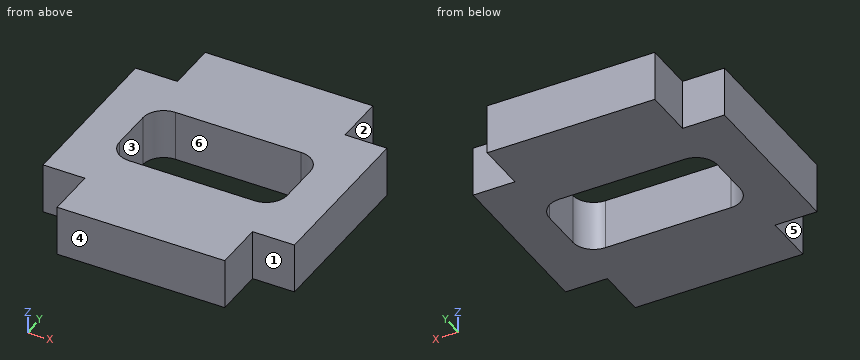
from build123d import *

# Parameters (mm, degrees)
SALIENTE_EXTRUIR1_DEPTH = 3


with BuildPart() as part:
    # Croquis1 → Saliente-Extruir1 (new body)
    with BuildSketch(Plane.XY):
        Polygon((-5, -8), (5, -8), (5, -5), (7.5, -5), (7.5, 5), (5, 5), (5, 8), (-5, 8), (-5, 5), (-7.5, 5), (-7.5, -5), (-5, -5), align=None)
        with BuildLine():
            ThreePointArc((5, -1.25), (4.633883476, -2.133883476), (3.75, -2.5))
            Line((3.75, -2.5), (-3.75, -2.5))
            ThreePointArc((-3.75, -2.5), (-4.633883476, -2.133883476), (-5, -1.25))
            Line((-5, -1.25), (-5, 1.25))
            ThreePointArc((-5, 1.25), (-4.633883476, 2.133883476), (-3.75, 2.5))
            Line((-3.75, 2.5), (3.75, 2.5))
            ThreePointArc((3.75, 2.5), (4.633883476, 2.133883476), (5, 1.25))
            Line((5, 1.25), (5, -1.25))
        make_face(mode=Mode.SUBTRACT)
    extrude(amount=SALIENTE_EXTRUIR1_DEPTH)


solid = part.part
Can you work these out from the model? Positions are in its coordinate system, mm. Face numbers are marked on the shaded views. A direction names the side the tool comes from. Coordinates: 2 decimals unless noted, no trailing zeros. Write each loop counter-clockwise with the first axis right and the second up, starting at its lowest first coordinate (ties: lowest second). Pieces come first, ordered by that corner, then holes. Notation, with made-up numbers: (-11, 83) -> (46, 83) arc R19 cw to (46, 92) -> close; hole circle Ø6 at (35, 8). An arc over 180 degrees is marked (long way). Write each question's results on one line, items separated by ' | '. Start each with the question number.
Item 1: If we section it at A-A, the plane x = 4.5: Write out the boundary of the cut face in (y, z).
Item 2: If we section it at B-B, the plane z = 2.3: Write out the boundary of the cut face in (x, y), and give its area (3 significant figures).
Item 3: If we section it at D-D, the plane y = -5.75: Write out the boundary of the cut face in (x, z), and give its area (3 significant figures).
Item 4: I'm going to push flat-ended pins straight in: P1, Ø0.9, axis at y = 6.5, z = 1.5, coming from the +X side; P2, Ø0.8, axis at x = 7, z = 2, coming from the -Y side; P3, Ø1.5, axis at y = 6.5, z = 1, coming from the -X side. Where does each tip first touch, or does it pass through?
Item 5: Please list where these lines run through material, in increasing order: probe 1 along Y at (x, z) = (-2, 0.3); probe 2 along Y at (x, z) = (-5.75, 0.5).
Item 6: On a 3-axis mill with a long thin cutter (end or side, diameter ignored), from which of +Z, -Z, +X, -X, +Y, -Y can I reach the whole of each face in a straight line? I mean the marked faces 1, 2 and 3. Say none if no direction works.
Item 7: If we section it at C-C, the plane y = 1: Write out the boundary of the cut face in (x, z), and give its area (3 significant figures).
Item 8: Thinking about a two-plate mould opening in Y: for the marked faces 4, 5 and 6, which applies, released by +Y, released by -Y, zero draft, split by the parting line, or undercut?
Answer block:
1) outline: (-8, 0) -> (-2.25, 0) -> (-2.25, 3) -> (-8, 3) -> close; (2.25, 0) -> (8, 0) -> (8, 3) -> (2.25, 3) -> close
2) outline: (-7.5, -5) -> (-5, -5) -> (-5, -8) -> (5, -8) -> (5, -5) -> (7.5, -5) -> (7.5, 5) -> (5, 5) -> (5, 8) -> (-5, 8) -> (-5, 5) -> (-7.5, 5) -> close; hole (-5, -1.25) arc R1.25 ccw to (-3.75, -2.5) -> (3.75, -2.5) arc R1.25 ccw to (5, -1.25) -> (5, 1.25) arc R1.25 ccw to (3.75, 2.5) -> (-3.75, 2.5) arc R1.25 ccw to (-5, 1.25) -> close | area: 161 mm²
3) outline: (-5, 0) -> (5, 0) -> (5, 3) -> (-5, 3) -> close | area: 30.0 mm²
4) P1: x = 5 | P2: y = -5 | P3: x = -5
5) probe 1: -8 to -2.5, 2.5 to 8 | probe 2: -5 to 5
6) face 1: +Z, -Z, +X, -Y | face 2: +Z, -Z, +X, +Y | face 3: +Z, -Z
7) outline: (-7.5, 0) -> (-5, 0) -> (-5, 3) -> (-7.5, 3) -> close; (5, 0) -> (7.5, 0) -> (7.5, 3) -> (5, 3) -> close | area: 15.0 mm²
8) face 4: released by -Y | face 5: zero draft | face 6: undercut
